Study the drawing (mm; zero at the part's minimum x, y, z) and answer. Coordinates: 2 decimals unless noted, no trailing zeros. Loops run counter-clockwise (first coordinate to the right, second up) from the corner with the lowest first, then second, coordinate; pieces in that order, holes last. Notation, with made-up numbers: (-18, 33.5) - (14, 33.5) arc R13 ccw to (14, 55.5) - close; hole circle Ø9 at (32.25, 18). An arc over 180 degrees is marked (long way). Put each result on its own line as item: value.
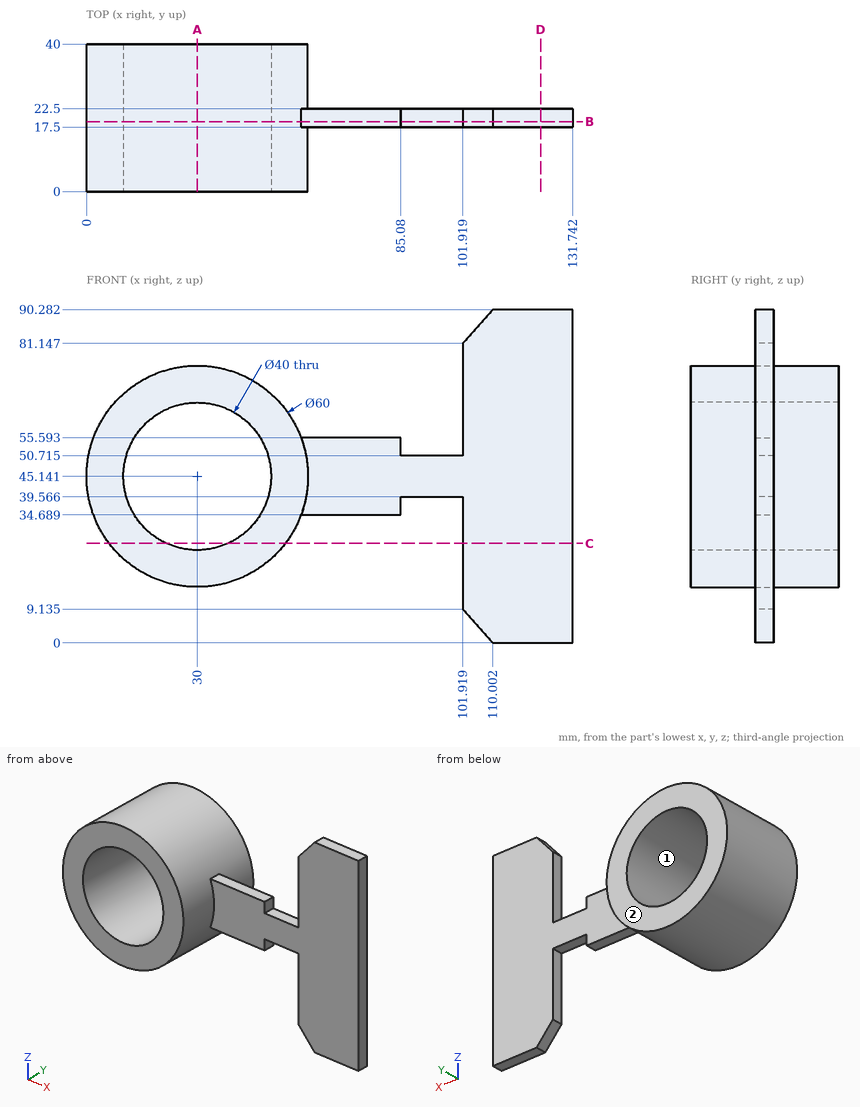
1) The part is cut by section B-B (y = 19). Give the vertices of the cut face in (x, z) (1 decimal), and give its area (3 significant figures).
Found:
outline: (58.1, 34.7) - (85.1, 34.7) - (85.1, 39.6) - (101.9, 39.6) - (101.9, 9.1) - (110, 0) - (131.7, 0) - (131.7, 90.3) - (110, 90.3) - (101.9, 81.1) - (101.9, 50.7) - (85.1, 50.7) - (85.1, 55.6) - (58.1, 55.6) arc R30 ccw (long way) to start; hole circle Ø40 at (30, 45.1)
area: 4,910 mm^2
2) Straight lines are drawn through the part: L1, parallel to Y at x = 73, z = 51; L2, parallel to X at y = 11, z = 42 (1 decimal); L3, parallel to X at y = 15, z = 50 (1 decimal). For each, find the intervals that lie inside material, in ascending order. Write a range as [from, to].
Found:
L1: y = [17.5, 22.5]
L2: x = [0.2, 10.2], [49.8, 59.8]
L3: x = [0.4, 10.6], [49.4, 59.6]
3) For a pull along X with two mould halves and no side action, classify the marked faces 1 and 2 as pulls with the +X half, pulls with the -X half, needs draft (parallel to the pull), parting line crosses it, or undercut.
Found:
face 1: undercut
face 2: needs draft
4) Each of these flat-tipped pins is pushed along its axis until it touches: pin 1 (3 mm diameter, centred on x = 108.5, z = 21, fed in from -Y); pin 2 (5.5 mm diameter, centred on x = 94.5, y = 20, fed in from -Z); pin 3 (5 mm diameter, centred on y = 11.5, z = 56.5, fed in from +X); pin 4 (12 mm diameter, centred on x = 23.5, z = 29, fed in from -Y). Where does it stop, or does it pass through?
Found:
pin 1: stops at y = 17.5
pin 2: stops at z = 39.57
pin 3: stops at x = 58.66
pin 4: stops at y = 0
5) The part is cut by section D-D (x = 123). Give the vertices of the cut face in (y, z).
Found:
outline: (17.5, 0) - (22.5, 0) - (22.5, 90.28) - (17.5, 90.28) - close
6) The part is cut by section A-A (x = 30). Give the vertices of the cut face in (y, z).
Found:
outline: (0, 15.14) - (40, 15.14) - (40, 25.14) - (0, 25.14) - close; (0, 65.14) - (40, 65.14) - (40, 75.14) - (0, 75.14) - close
7) The part is cut by section C-C (z = 27). Give the vertices of the cut face in (x, y), and give its area (3 significant figures).
Found:
outline: (6.11, 0) - (21.58, 0) - (21.58, 40) - (6.11, 40) - close; (38.42, 0) - (53.89, 0) - (53.89, 40) - (38.42, 40) - close; (101.92, 17.5) - (131.74, 17.5) - (131.74, 22.5) - (101.92, 22.5) - close
area: 1,390 mm^2
